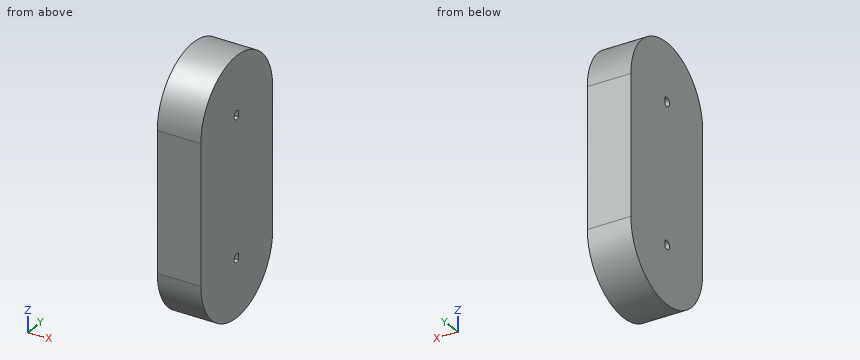
Autodesk Inventor part; units mm, degrees
ref_plane "YZ Plane" through (0, 0, 0) normal (1, 0, 0) x (0, 1, 0)
ref_plane "XZ Plane" through (0, 0, 0) normal (0, 1, 0) x (-1, 0, 0)
ref_plane "XY Plane" through (0, 0, 0) normal (0, 0, 1) x (1, 0, 0)
sketch "Szkic1" plane through (0, 0, 0) normal (1, 0, 0) x (0, 1, 0)
  line L0 (0, -24) -> (0, 24)
  circle A0 centre (20, 24) radius 20
  circle A1 centre (20, -24) radius 20
  line L1 (40, 24) -> (40, -24)
  line L2 (0, -24) -> (0, 24)
  point P0 (0, 0)
  dimension "d0" = 24
  dimension "d1" = 48
  dimension "d2" = 40
extrude "Wyciągnięcie proste1" add sketch "Szkic1" along normal blind 15 contours A1 | A0
sketch "Szkic2" plane through (15, 20, -24) normal (1, 0, 0) x (0, 0, -1)
  circle A0 centre (0, 0) radius 20
  line L0 (0, -20) -> (-48, -20)
  circle A1 centre (-48, 0) radius 20
  line L1 (0, 20) -> (-48, 20)
  line L2 (-48, 20) -> (-48, -20)
  line L3 (0, 20) -> (0, -20)
  point P0 (-24, -20)
extrude "Wyciągnięcie proste2" add sketch "Szkic2" against normal blind 15 contours A0 L0 A1 L1
sketch "Szkic3" plane through (15, 0, 0) normal (1, 0, 0) x (0, 0, -1)
  line L0 (0, 0) -> (0, 20)
  line L1 (-24, 40) -> (24, 40)
  line L2 (0, 20) -> (24, 20)
  line L3 (24, 20) -> (-24, 20)
  arc A0 (22.882, 21) -> (25.118, 21) centre (24, 20) ccw
  arc A1 (-25.118, 21) -> (-22.882, 21) centre (-24, 20) ccw
  line L4 (-24, 18.5) -> (-24, 21)
  line L5 (-24, 21) -> (-22.882, 21)
  line L6 (-24, 21) -> (-25.118, 21)
  line L7 (24, 18.5) -> (24, 21)
  line L8 (24, 21) -> (25.118, 21)
  line L9 (24, 21) -> (22.882, 21)
  dimension "d7" = 20
  dimension "d8" = 24
  dimension "d9" = 48
  dimension "d10" = 3
  dimension "d11" = 3
  dimension "d12" = 2.5
  dimension "d13" = 2.5
hole "Otwór1" at (15, 20, 24) direction (-1, 0, 0) diameter 3 end through all
sketch "Szkic4" plane through (15, 0, 0) normal (1, 0, 0) x (0, 0, -1)
  circle A0 centre (-24, 20) radius 1.5
  line L0 (-24, 20) -> (24, 20)
  point P0 (0, 0)
  dimension "d21" = 48
hole "Otwór2" at (15, 20, -24) direction (-1, 0, 0) diameter 3 end through all
sketch "Szkic5" plane through (15, 0, 0) normal (1, 0, 0) x (0, 0, -1)
  circle A0 centre (-24, 20) radius 1.5
  line L0 (-24, 18.5) -> (-24, 21)
  line L1 (-24, 21) -> (-22.882, 21)
  line L2 (-24, 21) -> (-25.118, 21)
  circle A1 centre (24, 20) radius 1.5
  line L3 (24, 18.5) -> (24, 21)
  line L4 (24, 21) -> (25.118, 21)
  line L5 (24, 21) -> (22.882, 21)
  point P0 (0, 0)
  dimension "d29" = 2.5
  dimension "d30" = 2.5
extrude "Wyciągnięcie proste3" add sketch "Szkic5" against normal blind 15 contours L1 L2 A0 | L4 L5 A1
properties part number "gasienice"
Can you work these out from the model? Positions are in its coordinate system, mm. Coordinates: 2 decimals unless noted, no trailing zeros. Write each loop counter-clockwise with the first axis right and the second up, starting at its lowest first coordinate (ties: lowest second). Pieces come first, ordered by that corner, then holes. Notation, with made-up numbers: (54, 73.25) -> (78, 73.25) arc R23 cw to (78, 81.25) -> close; hole circle Ø4 at (26, 22). An arc over 180 degrees is marked (long way). Answer as CSV lines item,"result".
1) If we section it at C-C on y = 14: Please give me the cut outline in (x, z).
Check result:
outline,"(0, -43.08) -> (15, -43.08) -> (15, 43.08) -> (0, 43.08) -> close"
2) Will these pins go through, and if not, where does the flat tip stop? P1, Ø2, axis at y = 6, z = 15, coming from the -X side; P2, Ø1, axis at x = 13, y = 26.5, coming from the +Z side.
Check result:
P1,"x = 0"
P2,"z = 43.08"
3) If we section it at A-A on y = 20: Please give me the cut outline in (x, z).
Check result:
outline,"(0, -44) -> (15, -44) -> (15, -25.5) -> (0, -25.5) -> close; (0, -22.5) -> (15, -22.5) -> (15, 22.5) -> (0, 22.5) -> close; (0, 25.5) -> (15, 25.5) -> (15, 44) -> (0, 44) -> close"
4) If we section it at B-B on x = 7: Please give me the cut outline in (y, z), then the cut area to 3 significant figures.
Check result:
outline,"(0, -24) arc R20 ccw to (40, -24) -> (40, 24) arc R20 ccw to (0, 24) -> close; hole (21, -25.12) -> (21, -22.88) arc R1.5 ccw (long way) to start; hole (21, 22.88) -> (21, 25.12) arc R1.5 ccw (long way) to start"
area,"3,160 mm²"
5) If I drill on line 1 (Z direction, x = 10.25, y = 20); line 2 (Y direction, x = 6.5, z = -24); line 3 (Z direction, x = 9.75, y = 20.5), over which ranges is the centre line in solid material (lowest first)? Write a range as from..to.
Check result:
line 1,"-44..-25.5, -22.5..22.5, 25.5..44"
line 2,"0..18.5, 21..40"
line 3,"-43.99..-25.41, -22.59..22.59, 25.41..43.99"
